Print and shaded views of the part. All mm, measured from the part's lowest x, y and z. A direction names the side the tool comes from. Coordinates: 2 decimals unless noted, no trailing zeros. Loops run counter-clockwise (first coordinate to the right, second up) from the corner with the lowest first, then second, coordinate; pieces in that order, holes last. Notation, with made-up numbers: M 88,77.5 L 112,77.5 A25 cw 112,113.5 Z; hole C -13.5,18 d7. An arc over 180 degrees is marked long. Use a Markdown table: item, result. Add a question column.
1) Band-saw the part on D-D (z = 5.25). List the corners of the cut face in (x, y), plus the area to 3 significant figures.
2) Band-saw the part on A-A (x = 3). List the corners of the cut face in (y, z).
3) Pull direction Y, two halves, no side cores. Call the marked faces 3, 4, 5 and 6: released by +Y, released by -Y, zero draft, split by the parting line, or undercut.
4) Pin check, flat tip, straight feed: pin 1 Ø2 at (x, y) = (1, 4.5) entering from +Z. Stop position of the tip, or through.
5) Band-saw the part on C-C (x = 5.25). List the corners of the cut face in (y, z).
6) Band-saw the part on B-B (y = 3.5). List the corners of the cut face in (x, z), plus the area to 3 significant figures.
7) Tool access for the marked faces 1 and 2: list every direction of +Z, -Z, +X, -X, +Y, -Y with a clear straight run to the whole face (end or side of a thin tool).
8) Wall check: probe 1 along Y at (x, z) = (1, 3.75); probe 2 along Z at (x, y) = (1.5, 8.5). Give the ranges that are in metal, low to high. Write a range as from..to.
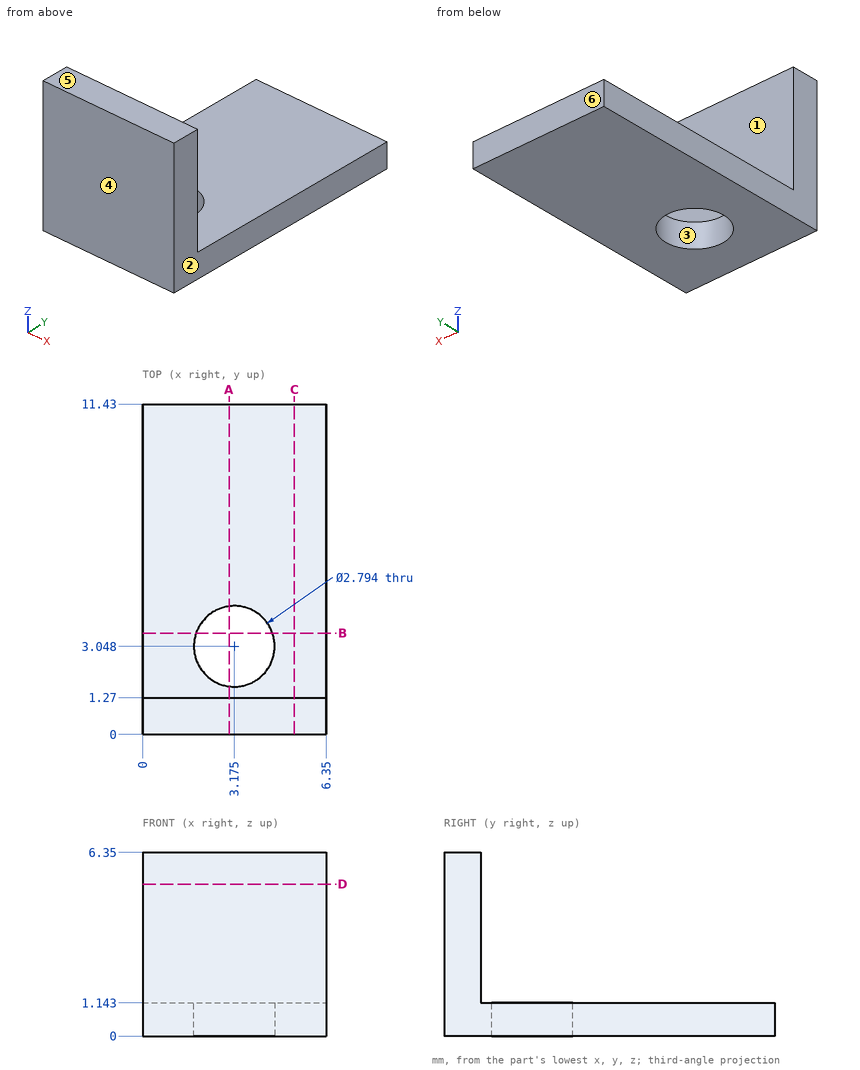
Entries:
| question | item | result |
|---|---|---|
| 1 | outline | M 0,0 L 6.35,0 L 6.35,1.27 L 0,1.27 Z |
| 1 | area | 8.06 mm2 |
| 2 | outline | M 0,0 L 1.66,0 L 1.66,1.14 L 1.27,1.14 L 1.27,6.35 L 0,6.35 Z; M 4.43,0 L 11.43,0 L 11.43,1.14 L 4.43,1.14 Z |
| 3 | face 3 | undercut |
| 3 | face 4 | released by -Y |
| 3 | face 5 | zero draft |
| 3 | face 6 | released by +Y |
| 4 | pin 1 | z = 1.14 |
| 5 | outline | M 0,0 L 11.43,0 L 11.43,1.14 L 1.27,1.14 L 1.27,6.35 L 0,6.35 Z |
| 6 | outline | M 0,0 L 1.85,0 L 1.85,1.14 L 0,1.14 Z; M 4.5,0 L 6.35,0 L 6.35,1.14 L 4.5,1.14 Z |
| 6 | area | 4.24 mm2 |
| 7 | face 1 | +Z, +X, -X, +Y |
| 7 | face 2 | +Z, -Z, +X, +Y, -Y |
| 8 | probe 1 | 0..1.27 |
| 8 | probe 2 | 0..1.14 |
